Autodesk Inventor part; units mm, degrees
ref_plane "YZ Plane" through (0, 0, 0) normal (1, 0, 0) x (0, 1, 0)
ref_plane "XZ Plane" through (0, 0, 0) normal (0, 1, 0) x (-1, 0, 0)
ref_plane "XY Plane" through (0, 0, 0) normal (0, 0, 1) x (1, 0, 0)
sketch "스케치1" plane through (0, 0, 0) normal (0, 0, 1) x (1, 0, 0)
  line L0 (-12.5, -12.5) -> (12.5, -12.5)
  line L1 (12.5, -12.5) -> (12.5, 12.5)
  line L2 (12.5, 12.5) -> (-12.5, 12.5)
  line L3 (-12.5, 12.5) -> (-12.5, -12.5)
  line L4 (-12.5, -12.5) -> (12.5, 12.5) construction
  line L5 (12.5, -12.5) -> (-12.5, 12.5) construction
  point P0 (0, 0)
  dimension "d0" = 25
  dimension "d1" = 25
extrude "돌출1" add sketch "스케치1" along normal blind 10.5
sketch "스케치2" plane through (0, 0, 10.5) normal (0, 0, 1) x (1, 0, 0)
  circle A0 centre (0, 0) radius 12
  dimension "d5" = 24
extrude "돌출2" cut sketch "스케치2" against normal blind 10
sketch "스케치3" plane through (0, 0, 0.5) normal (0, 0, 1) x (1, 0, 0)
  circle A0 centre (0, 0) radius 5
  line L0 (-0.9958, 12.5064) -> (1.0042, 12.5064)
  line L1 (1.0042, 12.5064) -> (1.0042, 1.749)
  line L2 (1.0042, 1.749) -> (-0.9958, 1.749)
  line L3 (-0.9958, 1.749) -> (-0.9958, 12.5064)
  line L4 (-0.9958, 12.5064) -> (1.0042, 1.749) construction
  line L5 (1.0042, 12.5064) -> (-0.9958, 1.749) construction
  line L6 (-10.333, -7.1156) -> (-11.333, -5.3835)
  line L7 (-11.333, -5.3835) -> (-2.0168, -0.0048)
  line L8 (-2.0168, -0.0048) -> (-1.0168, -1.7369)
  line L9 (-1.0168, -1.7369) -> (-10.333, -7.1156)
  line L10 (-10.333, -7.1156) -> (-2.0168, -0.0048) construction
  line L11 (-11.333, -5.3835) -> (-1.0168, -1.7369) construction
  line L12 (11.3288, -5.3908) -> (10.3288, -7.1229)
  line L13 (10.3288, -7.1229) -> (1.0126, -1.7442)
  line L14 (1.0126, -1.7442) -> (2.0126, -0.0121)
  line L15 (2.0126, -0.0121) -> (11.3288, -5.3908)
  line L16 (11.3288, -5.3908) -> (1.0126, -1.7442) construction
  line L17 (10.3288, -7.1229) -> (2.0126, -0.0121) construction
  circle A1 centre (0, 0) radius 12
  point P0 (0.0042, 7.1277)
  point P1 (-6.1749, -3.5602)
  point P2 (6.1707, -3.5675)
  point P3 (10.8544, -5.1169)
  point P4 (1.0042, 11.9579)
  point P5 (1.0042, 4.8981)
  point P6 (4.7413, -1.5875)
  point P7 (-9.8586, -6.8417)
  point P8 (9.8537, -6.8486)
  point P9 (3.7398, -3.3187)
  point P10 (-3.7455, -3.3123)
  point P11 (-0.9958, 11.9586)
  point P12 (-10.858, -5.1093)
  point P13 (-4.744, -1.5794)
  point P14 (-0.9958, 4.8998)
  dimension "d8" = 10
  dimension "d11" = 360
  dimension "d13" = 2
extrude "돌출3" cut sketch "스케치3" against normal blind 10 contours A0 L1 A1 L15 | A0 L7 A1 L3 | L13 A1 L9 A0
properties part number "쿨러"
Build history of the part. All positions in model axes, mm. A direction names the side the tool comes from. Round coordinates to 2 decimals unless told otherwise and drop trailing zeros. Write each loop counter-clockwise with the first axis right and the second up, starting at its lowest first coordinate (ties: lowest second). Pieces come first, ordered by that corner, then holes. Notation, with made-up numbers: (2.5, 57.25) -> (35.5, 57.25) arc R28 cw to (35.5, 92.25) -> close; hole circle Ø1 at (44, 9.25). An arc over 180 degrees is marked (long way). Write item = value, one per line.
(1) Band-saw the part on C-C (x = -7.5). Give the cut face in (y, z).
Answer:
outline = (-12.5, 0) -> (-9.37, 0) -> (-9.37, 10.5) -> (-12.5, 10.5) -> close; (-5.48, 0) -> (-3.17, 0) -> (-3.17, 0.5) -> (-5.48, 0.5) -> close; (9.37, 0) -> (12.5, 0) -> (12.5, 10.5) -> (9.37, 10.5) -> close
(2) Probe L1, parallel to Y at x = 0, z = 2.75; L2, parallel to Y at x = 2, z = 2. List the from-to ranges inside material, lowest first.
Answer:
L1 = -12.5 to -12, 12 to 12.5
L2 = -12.5 to -11.83, 11.83 to 12.5
(3) Band-saw the part on B-B (y = 0). Give the cut face in (x, z), then the cut area to 3 significant figures.
Answer:
outline = (-12.5, 0) -> (-12, 0) -> (-12, 10.5) -> (-12.5, 10.5) -> close; (-5, 0) -> (5, 0) -> (5, 0.5) -> (-5, 0.5) -> close; (12, 0) -> (12.5, 0) -> (12.5, 10.5) -> (12, 10.5) -> close
area = 15.5 mm2
(4) Two-plate mould, pull along Y, no slides. Class faces 4 (the face through (4.362, 2.445, 0.254)), 5 (the face through (0, 12.5, 5)), 6 (the face through (-7, -10, 10.5)): pulls with the +Y half, pulls with the -Y half, needs draft (parallel to the pull), parting line crosses it, or undercut.
Answer:
face_4 = undercut
face_5 = pulls with the +Y half
face_6 = needs draft
(5) Flat gauge pin, fed straight in: pin 1 (8 mm diameter, centred on x = -5.5, y = -1.5, fed in from +Z). Where does the tip first touch, or does it go through?
Answer:
pin_1 = 0.5
(6) Tool access for faces 1 (the face through (0, 0, 0.5)), 2 (the face through (-7.844, -3.369, 0.254)), 3 (the face through (-12.5, 0, 5)): list every direction of +Z, -Z, +X, -X, +Y, -Y with a clear straight run to the whole face (end or side of a thin tool).
Answer:
face_1 = +Z
face_2 = +Z, -Z
face_3 = +Z, -Z, -X, +Y, -Y
(7) Band-saw the part on D-D (z = 2). Give the cut face in (x, y).
Answer:
outline = (-12.5, -12.5) -> (12.5, -12.5) -> (12.5, 12.5) -> (-12.5, 12.5) -> close; hole circle Ø24 at (0, 0)
(8) Band-saw the part on A-A (x = 0). Give the cut face in (y, z).
Answer:
outline = (-12.5, 0) -> (-12, 0) -> (-12, 10.5) -> (-12.5, 10.5) -> close; (-5, 0) -> (12.5, 0) -> (12.5, 10.5) -> (12, 10.5) -> (12, 0.5) -> (-5, 0.5) -> close
